Autodesk Inventor part; units mm, degrees
ref_plane "YZ Plane" through (0, 0, 0) normal (1, 0, 0) x (0, 1, 0)
ref_plane "XZ Plane" through (0, 0, 0) normal (0, 1, 0) x (-1, 0, 0)
ref_plane "XY Plane" through (0, 0, 0) normal (0, 0, 1) x (1, 0, 0)
sketch "Sketch1" plane through (0, 0, 0) normal (0, 1, 0) x (-1, 0, 0)
  line L0 (94.0269, 81.28) -> (27.9869, 81.28)
  line L1 (94.0269, -81.28) -> (27.9869, -81.28)
  line L2 (94.0269, 81.28) -> (122.0139, 0)
  line L3 (94.0269, 81.28) -> (179.9904, 81.28) construction
  line L4 (122.0139, 0) -> (94.0269, -81.28)
  line L5 (27.9869, 81.28) -> (0, 0)
  line L6 (27.9869, 81.28) -> (113.9504, 81.28) construction
  line L7 (0, 0) -> (27.9869, -81.28)
  dimension "d6" = 66.04
  dimension "d7" = 162.56
  dimension "d8" = 71
  dimension "d9" = 109
  dimension "d10" = 109
extrude "Extrusion1" add sketch "Sketch1" along normal blind 12.7
fillet "Fillet1" radius 8.89 6 edges at (-27.9869, 6.35, 81.28) (-94.0269, 6.35, 81.28) (0, 6.35, 0) (-27.9869, 6.35, -81.28) (-122.0139, 6.35, 0) (-94.0269, 6.35, -81.28)
sketch "Sketch4" plane through (0, 0, 0) normal (0, -1, 0) x (1, 0, 0)
  line L0 (-52.8789, 81.28) -> (-69.1349, 81.28)
  line L1 (-69.1349, 81.28) -> (-69.1349, 64.135)
  line L2 (-65.9599, 60.96) -> (-56.0539, 60.96)
  line L3 (-52.8789, 64.135) -> (-52.8789, 81.28)
  line L4 (-87.6858, 81.28) -> (-34.3281, 81.28)
  arc A0 (-56.0539, 60.96) -> (-52.8789, 64.135) centre (-56.0539, 64.135) ccw
  arc A1 (-69.1349, 64.135) -> (-65.9599, 60.96) centre (-65.9599, 64.135) ccw
  point P0 (0, 0)
  point P1 (-69.1349, 60.96)
  point P2 (-52.8789, 60.96)
  point P3 (-61.0069, 81.28)
  dimension "d28" = 16.256
  dimension "d29" = 20.32
  dimension "d32" = 3.175
extrude "Extrusion4" cut sketch "Sketch4" against normal blind 4.445
mirror "Mirror2" about plane through (0, 0, 0) normal (0, 0, 1) of "Extrusion4"
Geometry check sheet. Reference: the model listing, model coordinates, mm. A direction names the side the tool comes from. Coordinates: 2 decimals unless noted, no trailing zeros. Order: outer loops, then holes, each group sorted by start corner. A loop starts at its lowest first (then second) coordinate and runs counter-clockwise, first axis right, second up. Notation, with made-up numbers: M 34.25,62 L 42.25,62 A5 ccw 42.25,68 Z; hole C -14.5,-35.75 d5. An arc over 180 degrees is marked long. Answer as a JSON object with one key per item and string values.
Q1. Tool access check on faces 1 (the flat face through (-108.73, 6.26, -38.58)), 2 (the flat face through (-69.135, 2, -73)), 3 (the flat face through (-69.135, 2, 73)). Record the directions out of +Z, -Z, +X, -X, +Y, -Y that give a thin tool (end or side, any length) a straight path to the whole face; none if there is none.
Results are:
{"face 1": "-Z, -X, +Y, -Y", "face 2": "-Z, -Y", "face 3": "+Z, -Y"}
Q2. Scan lines: line 1 (Y direction, x = -67, z = -64.5) (3 decimals); line 2 (X direction, y = 6.75, z = -29); line 3 (X direction, y = 3.25, z = 33). Record each from-to range of solid material in increasing order.
Results are:
{"line 1": "y = 4.445 to 12.7", "line 2": "x = -112.03 to -9.99", "line 3": "x = -110.65 to -11.36"}
Q3. Cross-section at A-A on y = 10.25. Record the cut outline in (x, z).
Results are:
{"outline": "M -121.02,-2.89 L -96.09,-75.28 A8.89 ccw -87.69,-81.28 L -34.33,-81.28 A8.89 ccw -25.92,-75.28 L -1,-2.89 A8.89 ccw -1,2.89 L -25.92,75.28 A8.89 ccw -34.33,81.28 L -87.69,81.28 A8.89 ccw -96.09,75.28 L -121.02,2.89 A8.89 ccw Z"}
Q4. Cross-section at D-D on y = 2.25. Record the cut outline in (x, z) (3 decimals), and give its area (3 significant figures).
Results are:
{"outline": "M -121.017,-2.894 L -96.091,-75.284 A8.89 ccw -87.686,-81.28 L -69.135,-81.28 L -69.135,-64.135 A3.175 cw -65.96,-60.96 L -56.054,-60.96 A3.175 cw -52.879,-64.135 L -52.879,-81.28 L -34.328,-81.28 A8.89 ccw -25.922,-75.284 L -0.997,-2.894 A8.89 ccw -0.997,2.894 L -25.922,75.284 A8.89 ccw -34.328,81.28 L -52.879,81.28 L -52.879,64.135 A3.175 cw -56.054,60.96 L -65.96,60.96 A3.175 cw -69.135,64.135 L -69.135,81.28 L -87.686,81.28 A8.89 ccw -96.091,75.284 L -121.017,2.894 A8.89 ccw Z", "area": "14,600 mm²"}
Q5. Cross-section at B-B on z = -70.5. Record the cut outline in (x, y) (3 decimals).
Results are:
{"outline": "M -97.739,0 L -69.135,0 L -69.135,4.445 L -52.879,4.445 L -52.879,0 L -24.275,0 L -24.275,12.7 L -97.739,12.7 Z"}
Q6. Depth check by flat-ended pin: pin 1 Ø5 at (y, z) = (1.5, 43) entering from -X; pin 2 Ø3 at (y, z) = (4.5, -54.5) entering from -X; pin 3 Ø2 at (y, z) = (2, 77) entering from +X. Enter the tip coordinate at first touch or a pass-through.
Results are:
{"pin 1": "stops at x = -108.07", "pin 2": "stops at x = -103.76", "pin 3": "stops at x = -26.2"}
Q7. Release check for a two-part mould opening along X. For faces 4 (the flat face through (-13.285, 6.261, -38.583)), 5 (the flat face through (-52.879, 2, -73)), 6 (the cylindrical face through (-68.23, 2.191, 61.915)), 7 (the cylindrical face through (-121.5, 6.4, 0)) record: released by +X, released by -X, zero draft, split by the parting line, or undercut.
Results are:
{"face 4": "released by +X", "face 5": "undercut", "face 6": "undercut", "face 7": "released by -X"}
Q8. Cross-section at C-C on x = -10. Record the cut outline in (y, z), and give its area (3 significant figures).
Results are:
{"outline": "M 0,-29.04 L 12.7,-29.04 L 12.7,29.04 L 0,29.04 Z", "area": "738 mm²"}
